Geometry: final body of the model. Coordinates: model frame, mm. Face numbers are marked on the shaded views. Round coordinates to 2 decimals unless told otherwise and drop trailing zeros. Order: outer loops, then holes, each group sorted by start corner. A loop starts at its lowest first (then second) coordinate and runs counter-clockwise, first axis right, second up. Notation, with made-up numbers: (-2, 7) -> (24, 7) arc R16 cw to (24, 16) -> close; hole circle Ø7 at (-10.5, -37.75). An arc over 180 degrees is marked (long way). Put each result on its own line as item: value.
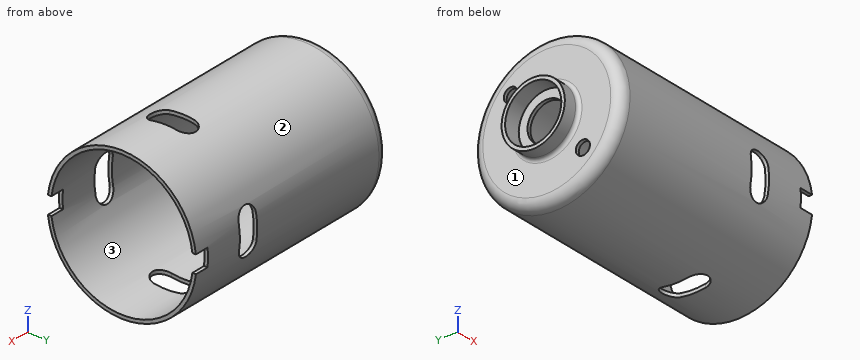
```python
from build123d import *

# Parameters (mm, degrees)
CUT_EXTRUDE6_REACH      = 87.122
CUT_EXTRUDE6_END_RADIUS = 20.2
CIRPATTERN21_COUNT      = 4
SKETCH10_W              = 4
SKETCH10_H              = 5
CUT_EXTRUDE7_DEPTH      = 10
CIRPATTERN22_COUNT      = 2
CUT_EXTRUDE8_REACH      = 74.491
SKETCH13_R              = 2


with BuildPart() as part:
    # Sketch1 → Revolve2 (revolve)
    with BuildSketch(Plane.XY, mode=Mode.PRIVATE) as revolve2_sk:
        with BuildLine():
            Line((70.7, 21.2), (7.7, 21.2))
            ThreePointArc((7.7, 21.2), (5.578679656, 20.321320344), (4.7, 18.2))
            Line((4.7, 18.2), (4.7, 10))
            ThreePointArc((4.7, 10), (4.407106781, 9.292893219), (3.7, 9))
            Line((3.7, 9), (0, 9))
            Line((0, 9), (0, 8))
            Line((0, 8), (4.7, 8))
            Line((4.7, 8), (4.7, 5.5))
            Line((4.7, 5.5), (5.7, 5.5))
            Line((5.7, 5.5), (5.7, 8))
            Line((5.7, 8), (5.7, 18.2))
            ThreePointArc((5.7, 18.2), (6.285786438, 19.614213562), (7.7, 20.2))
            Line((7.7, 20.2), (70.7, 20.2))
            Line((70.7, 20.2), (70.7, 21.2))
        make_face()
    revolve(revolve2_sk.sketch.rotate(Axis((0, 0, 0), (1, 0, 0)), 90), axis=Axis((0, 0, 0), (1, 0, 0)))

    # Cut-Extrude6: up to this cylinder (the profile starts outside it)
    cut_extrude6_end = Plane(origin=(52.7, 0, 0), z_dir=(-1, 0, 0)) * Cylinder(CUT_EXTRUDE6_END_RADIUS, 215.644, mode=Mode.PRIVATE)
    # Sketch8 → Cut-Extrude6 (cut, up to the surface)
    with BuildSketch(Plane(origin=(70.7, 21.2, 0), x_dir=(1, 0, 0), z_dir=(0, 1, 0)), mode=Mode.PRIVATE) as cut_extrude6_sk1:
        with BuildLine():
            Line((-15, 3.153060045), (-15, -3.846939955))
            ThreePointArc((-15, -3.846939955), (-18, -6.846939955), (-21, -3.846939955))
            Line((-21, -3.846939955), (-21, 3.153060045))
            ThreePointArc((-21, 3.153060045), (-18, 6.153060045), (-15, 3.153060045))
        make_face()
    cut_extrude6_tool1 = extrude(cut_extrude6_sk1.sketch, amount=-CUT_EXTRUDE6_REACH, mode=Mode.PRIVATE) - cut_extrude6_end
    cut_extrude6 = cut_extrude6_tool1.solids().sort_by_distance((52.7, 21.2, 0.34694))[0]
    add(cut_extrude6, mode=Mode.SUBTRACT)

    # CirPattern21: Cut-Extrude6 ×4 about axis
    cirpattern21_axis = Axis((0, 0, 0), (-1, 0, 0))
    for i in range(1, CIRPATTERN21_COUNT):
        add(cut_extrude6.rotate(cirpattern21_axis, i * 360 / CIRPATTERN21_COUNT), mode=Mode.SUBTRACT)

    # Sketch10 → Cut-Extrude7 (cut)
    with BuildSketch(Plane(origin=(70.7, 21.2, 0), x_dir=(1, 0, 0), z_dir=(0, 1, 0))):
        with Locations((-2, 0)):
            Rectangle(SKETCH10_W, SKETCH10_H)
    cut_extrude7 = extrude(amount=-CUT_EXTRUDE7_DEPTH, mode=Mode.SUBTRACT)

    # CirPattern22: Cut-Extrude7 ×2 about axis
    cirpattern22_axis = Axis((0, 0, 0), (-1, 0, 0))
    for i in range(1, CIRPATTERN22_COUNT):
        add(cut_extrude7.rotate(cirpattern22_axis, i * 360 / CIRPATTERN22_COUNT), mode=Mode.SUBTRACT)

    # Sketch13 → Cut-Extrude8 (cut, up to next)
    with BuildSketch(Plane.ZY.offset(-4.7), mode=Mode.PRIVATE) as cut_extrude8_sk1:
        with Locations((10.253048327, 10.253048327)):
            Circle(SKETCH13_R)
    cut_extrude8_tool1 = extrude(cut_extrude8_sk1.sketch, amount=-CUT_EXTRUDE8_REACH, mode=Mode.PRIVATE) & part.part
    # Sketch13 → Cut-Extrude8 (cut, up to next)
    with BuildSketch(Plane.ZY.offset(-4.7), mode=Mode.PRIVATE) as cut_extrude8_sk2:
        with Locations((-10.253048327, -10.253048327)):
            Circle(SKETCH13_R)
    cut_extrude8_tool2 = extrude(cut_extrude8_sk2.sketch, amount=-CUT_EXTRUDE8_REACH, mode=Mode.PRIVATE) & part.part
    add(cut_extrude8_tool1.solids().sort_by_distance((4.7, 10.253048, 10.253048))[0], mode=Mode.SUBTRACT)
    add(cut_extrude8_tool2.solids().sort_by_distance((4.7, -10.253048, -10.253048))[0], mode=Mode.SUBTRACT)


solid = part.part
```
1. Cut plane A-A on y = 0. State how many separate pieces and enclosed holes the cut face has, and give its area (3 significant figures).
Ans:
separate pieces: 4
enclosed holes: 0
area: 157 mm²
2. Contact query for flat-ended pins moving along their axis: P1, Ø18, axis at y = 4.5, z = 9, coming from the +X side; P2, Ø1.1, axis at y = 1.5, z = 20.5, coming from the -X side; P3, Ø1.5, axis at x = 38.5, z = 12, coming from the -Y side. Output: stop coordinate, or through.
Ans:
P1: x = 5.9
P2: x = 5.3
P3: y = -17.97
3. Material intervals for probe 1 along Y at (x, z) = (2.55, 0); probe 2 along X at (y, z) = (5.5, -1); probe 3 along Z at (x, y) = (41, -10), sorted ascending.
Ans:
probe 1: -9 to -8, 8 to 9
probe 2: 4.7 to 5.7
probe 3: -18.69 to -17.55, 17.55 to 18.69
4. Cut plane D-D on x = 38. Return loops of the section in (y, z), and give its area (3 significant figures).
Ans:
outline: circle Ø42.4 at (0, 0); hole circle Ø40.4 at (0, 0)
area: 130 mm²
5. Cut plane C-C on x = 52.7. Return loops of the section in (y, z), and give its area (3 significant figures).
Ans:
outline: (-20.29, 6.15) -> (-19.24, 6.15) arc R20.2 cw to (-6.85, 19) -> (-6.85, 20.06) arc R21.2 ccw to start; (-20.06, -6.85) arc R21.2 ccw to (-6.15, -20.29) -> (-6.15, -19.24) arc R20.2 cw to (-19, -6.85) -> close; (6.15, 19.24) arc R20.2 cw to (19, 6.85) -> (20.06, 6.85) arc R21.2 ccw to (6.15, 20.29) -> close; (6.85, -20.06) arc R21.2 ccw to (20.29, -6.15) -> (19.24, -6.15) arc R20.2 cw to (6.85, -19) -> close
area: 77.2 mm²
6. Draft query along Z for the marked faces 1, 2 and 3. Return one class per face: +Z half, -Z half, draft (parallel to the pull), parting line (faces both ways), or undercut.
Ans:
face 1: draft
face 2: parting line
face 3: undercut
